For this review, take the finished solid that the model builds, in its own axes (mm). A direction names the side the tool comes from. Coordinates: 2 decimals unless noted, no trailing zeros. Loops run counter-clockwise (first coordinate to the right, second up) from the corner with the lowest first, then second, coordinate; pieces in that order, holes last. Notation, with made-up numbers: (32.25, 42.5) -> (37.25, 42.5) arc R20 ccw to (37.25, 58.5) -> close; hole circle Ø6 at (-1.5, -29.5). An arc over 180 degrees is marked (long way). One line per item, written item: value.
from build123d import *

# Parameters (mm, degrees)
F0_W      = 20
F0_H      = 20
F1_DEPTH  = 2
F3_DEPTH  = 10
F4_W      = 10
F4_H      = 4
F5_DEPTH  = 10
F6_R      = 1
F8_R      = 1.9
F9_DEPTH  = 25
F8_R_2    = 3.6
F10_DEPTH = 15
F11_SIZE  = 2


with BuildPart() as f1:
    # F0 (on Top) → F1 (new body, symmetric)
    with BuildSketch(Plane.XY):
        Rectangle(F0_W, F0_H)
    extrude(amount=F1_DEPTH, both=True)

    # F2 (on Right) → F3 (join, symmetric)
    with BuildSketch(Plane.YZ):
        with BuildLine():
            Line((0, 0), (6.6592096346, 0))
            ThreePointArc((6.6592096346, 0), (4.0870468344, 16.5868898597), (-10, 7.4602229888))
            Line((-10, 7.4602229888), (-10, 0))
            Line((-10, 0), (-6.6592096346, 0))
            Line((-6.6592096346, 0), (0, 0))
        make_face()
        with BuildLine():
            ThreePointArc((-4.3801786394, 2), (-3.0280975483, 13.7713738535), (7, 7.4602229888))
            ThreePointArc((7, 7.4602229888), (6.3111508648, 4.4321254404), (4.3801786394, 2))
            ThreePointArc((4.3801786394, 2), (0, 0.4602229888), (-4.3801786394, 2))
        make_face(mode=Mode.SUBTRACT)
    extrude(amount=F3_DEPTH, both=True)

    # F4 (on Right) → F5 (cut, symmetric)
    with BuildSketch(Plane.YZ):
        with Locations((7.6843140367, 4)):
            Rectangle(F4_W, F4_H)
    extrude(amount=F5_DEPTH, both=True, mode=Mode.SUBTRACT)

    # F6
    f6_edges = [f1.edges().sort_by_distance(p)[0] for p in [
        (0, 10, 2),
        (0, 9.892813, 6),
        (0, 6.846002, 6),
        (0, -4.380179, 2),
    ]]
    fillet(f6_edges, radius=F6_R)

    # F8 (on offset) → F9 (cut)
    with BuildSketch(Plane(origin=(0, 0, 20.2), x_dir=(1, 0, 0), z_dir=(0, 0, -1))):
        Circle(F8_R)
    extrude(amount=F9_DEPTH, mode=Mode.SUBTRACT)

    # F8 (on offset) → F10 (cut)
    with BuildSketch(Plane(origin=(0, 0, 20.2), x_dir=(1, 0, 0), z_dir=(0, 0, -1))):
        Circle(F8_R_2)
        Circle(F8_R, mode=Mode.SUBTRACT)
    extrude(amount=F10_DEPTH, mode=Mode.SUBTRACT)

    # F11
    f11_edges = [f1.edges().sort_by_distance(p)[0] for p in [
        (-1.9, 0, 2),
    ]]
    chamfer(f11_edges, length=F11_SIZE)


solid = f1.part
1. To check wall thickness, follow probe 1 along Y at (x, z) = (4.75, 7.75); probe 2 along Y at (x, z) = (0, -0.5); probe 3 along X at (y, z) = (0, 15.1). State the ranges of each line that lie inside material, in increasing order. Write a range as from..to.
Return value:
probe 1: y = -10..-6.99, 6.99..10
probe 2: y = -10..-1.9, 1.9..10
probe 3: x = -10..-3.6, 3.6..10
2. For faces 1 (the cylindrical face through (-1.9, -0.08, -0.99)), 2 (the cylindrical face through (0.14, 9.699, 1.715)), 3 (the cylindrical face through (0.14, 7.267, 6.305)), list the 3-axis set-ups (+Z, -Z, +X, -X, +Y, -Y) from which the entire face can be reached by the end or side of a thin tool; tool diameter is ignored.
Return value:
face 1: +Z, -Z
face 2: +X, -X, +Y
face 3: +X, -X
3. Take a section at A-A, the plane y = 0. Give the boundary of the cut face in (x, z).
Return value:
outline: (-10, -2) -> (-1.9, -2) -> (-1.9, 0) -> (-3.9, 2) -> (-10, 2) -> close; (-10, 14.46) -> (-3.6, 14.46) -> (-3.6, 17.46) -> (-10, 17.46) -> close; (1.9, -2) -> (10, -2) -> (10, 2) -> (3.9, 2) -> (1.9, 0) -> close; (3.6, 14.46) -> (10, 14.46) -> (10, 17.46) -> (3.6, 17.46) -> close
4. The part is to be moulded in two halves that separate along X. For faces 4 (the flat face through (0, 5, 2)), 5 (the cylindrical face through (1.661, 3.194, 15.493)), 6 (the flat face through (-10, 0, 1)), say which applies: pulls with the +X half, pulls with the -X half, needs draft (parallel to the pull), parting line crosses it, or undercut.
Return value:
face 4: needs draft
face 5: undercut
face 6: pulls with the -X half
5. Take a section at D-D, the plane z = 16. Give the boundary of the cut face in (x, y), and give its area (3 significant figures).
Return value:
outline: (-10, -5.2) -> (10, -5.2) -> (10, 5.2) -> (-10, 5.2) -> close; hole circle Ø7.2 at (0, 0)
area: 167 mm2
6. Insertion check: pin 1 Ø6 at (x, y) = (0, 0) entering from +Z; pin 2 Ø1.5 at (x, y) = (0.5, -4.5) entering from +Z; pin 3 Ø6.5 at (x, y) = (-1.5, 5.5) entering from +Z. Each pin has a flat end and moves straight along its axis. Give the tip position at first contact, or say it passes through.
Return value:
pin 1: stops at z = 1.1
pin 2: stops at z = 16.73
pin 3: stops at z = 17.15
7. Take a section at C-C, the plane y = 7.5. Give the boundary of the cut face in (x, z).
Return value:
outline: (-10, -2) -> (10, -2) -> (10, 2) -> (-10, 2) -> close; (-10, 6.13) -> (10, 6.13) -> (10, 14.07) -> (-10, 14.07) -> close
8. Take a section at B-B, the plane x = 0. Give the boundary of the cut face in (y, z), and give its area (3 significant figures).
Return value:
outline: (-10, -2) -> (-1.9, -2) -> (-1.9, 0) -> (-3.9, 2) -> (-4.01, 2) arc R1 cw to (-4.68, 2.26) arc R7 cw to (-3.6, 13.46) -> (-3.6, 16.79) arc R10 ccw to (-10, 7.46) -> close; (1.9, -2) -> (10, -2) -> (10, 1) arc R1 ccw to (9, 2) -> (3.9, 2) -> (1.9, 0) -> close; (3.6, 13.46) arc R7 cw to (6.99, 7.06) arc R1 ccw to (7.99, 6) -> (8.99, 6) arc R1 ccw to (9.99, 6.95) arc R10 ccw to (3.6, 16.79) -> close
area: 143 mm2
